```python
from build123d import *

# Parameters (mm, degrees)
EXTRUDE_START                           = -72
EXTRUDE_SKETCH_1_R                      = 82
EXTRUDE_SKETCH_1_R_2                    = 66
EXTRUDE_1_DEPTH                         = 12
EXTRUDE_START_2                         = -380
EXTRUDE_SKETCH_2_R                      = 3
EXTRUDE_2_DEPTH                         = 308
EXTRUDE_SKETCH_3_R                      = 3
EXTRUDE_3_DEPTH                         = 308
EXTRUDE_SKETCH_4_R                      = 3
EXTRUDE_4_DEPTH                         = 308
EXTRUDE_SKETCH_5_R                      = 3
EXTRUDE_5_DEPTH                         = 308
EXTRUDE_SKETCH_6_R                      = 3
EXTRUDE_6_DEPTH                         = 308
EXTRUDE_SKETCH_7_R                      = 3
EXTRUDE_7_DEPTH                         = 308
EXTRUDE_SKETCH_8_R                      = 3
EXTRUDE_8_DEPTH                         = 308
EXTRUDE_SKETCH_9_R                      = 3
EXTRUDE_9_DEPTH                         = 308
EXTRUDE_START_3                         = -170
EXTRUDE_SKETCH_10_R                     = 80
EXTRUDE_SKETCH_10_R_2                   = 70
EXTRUDE_10_DEPTH                        = 4
EXTRUDE_START_4                         = -275
EXTRUDE_SKETCH_11_R                     = 80
EXTRUDE_SKETCH_11_R_2                   = 70
EXTRUDE_11_DEPTH                        = 4
EXTRUDE_START_5                         = -384
EXTRUDE_SKETCH_12_R                     = 80
EXTRUDE_SKETCH_12_R_2                   = 64
EXTRUDE_12_DEPTH                        = 4
EXTRUDE_SKETCH_13_W                     = 129
EXTRUDE_SKETCH_13_H                     = 6
EXTRUDE_13_DEPTH                        = 4
EXTRUDE_SKETCH_14_W                     = 6
EXTRUDE_SKETCH_14_H                     = 61.49
EXTRUDE_14_DEPTH                        = 4
EXTRUDE_SKETCH_15_W                     = 6
EXTRUDE_SKETCH_15_H                     = 61.49
EXTRUDE_15_DEPTH                        = 4
COMBINE_START                           = -384
COMBINE_WELD_ASSEMBLY_OF_FEATURES_OUT_W = 6
COMBINE_WELD_ASSEMBLY_OF_FEATURES_OUT_H = 0.01
COMBINE_WELD_ASSEMBLY_OF_FEATURES_DEPTH = 4


# Read off the part's stored shape, not the designer's step: Combine _weld _ assembly of features_
with BuildPart() as part:
    # Extrude sketch 1 → Extrude 1 (new body)
    with BuildSketch(Plane.XY.offset(EXTRUDE_START)):
        with Locations((240, 0)):
            Circle(EXTRUDE_SKETCH_1_R)
        with Locations((240, 0)):
            Circle(EXTRUDE_SKETCH_1_R_2, mode=Mode.SUBTRACT)
    extrude(amount=EXTRUDE_1_DEPTH)


with BuildPart() as body_2:
    # Extrude sketch 2 → Extrude 2 (new body)
    with BuildSketch(Plane.XY.offset(EXTRUDE_START_2)):
        with Locations((308.367085406, 28.318573995)):
            Circle(EXTRUDE_SKETCH_2_R)
    extrude(amount=EXTRUDE_2_DEPTH)


with BuildPart() as body_3:
    # Extrude sketch 3 → Extrude 3 (new body)
    with BuildSketch(Plane.XY.offset(EXTRUDE_START_2)):
        with Locations((268.318573995, 68.367085406)):
            Circle(EXTRUDE_SKETCH_3_R)
    extrude(amount=EXTRUDE_3_DEPTH)


with BuildPart() as body_4:
    # Extrude sketch 4 → Extrude 4 (new body)
    with BuildSketch(Plane.XY.offset(EXTRUDE_START_2)):
        with Locations((211.681426005, 68.367085406)):
            Circle(EXTRUDE_SKETCH_4_R)
    extrude(amount=EXTRUDE_4_DEPTH)


with BuildPart() as body_5:
    # Extrude sketch 5 → Extrude 5 (new body)
    with BuildSketch(Plane.XY.offset(EXTRUDE_START_2)):
        with Locations((171.632914594, 28.318573995)):
            Circle(EXTRUDE_SKETCH_5_R)
    extrude(amount=EXTRUDE_5_DEPTH)


with BuildPart() as body_6:
    # Extrude sketch 6 → Extrude 6 (new body)
    with BuildSketch(Plane.XY.offset(EXTRUDE_START_2)):
        with Locations((171.632914594, -28.318573995)):
            Circle(EXTRUDE_SKETCH_6_R)
    extrude(amount=EXTRUDE_6_DEPTH)


with BuildPart() as body_7:
    # Extrude sketch 7 → Extrude 7 (new body)
    with BuildSketch(Plane.XY.offset(EXTRUDE_START_2)):
        with Locations((211.681426005, -68.367085406)):
            Circle(EXTRUDE_SKETCH_7_R)
    extrude(amount=EXTRUDE_7_DEPTH)



with BuildPart() as body_8:
    # Extrude sketch 8 → Extrude 8 (new body)
    with BuildSketch(Plane.XY.offset(EXTRUDE_START_2)):
        with Locations((268.318573995, -68.367085406)):
            Circle(EXTRUDE_SKETCH_8_R)
    extrude(amount=EXTRUDE_8_DEPTH)


with BuildPart() as body_9:
    # Extrude sketch 9 → Extrude 9 (new body)
    with BuildSketch(Plane.XY.offset(EXTRUDE_START_2)):
        with Locations((308.367085406, -28.318573995)):
            Circle(EXTRUDE_SKETCH_9_R)
    extrude(amount=EXTRUDE_9_DEPTH)


with BuildPart() as body_10:
    # Extrude sketch 10 → Extrude 10 (new body)
    with BuildSketch(Plane.XY.offset(EXTRUDE_START_3)):
        with Locations((240, 0)):
            Circle(EXTRUDE_SKETCH_10_R)
        with Locations((240, 0)):
            Circle(EXTRUDE_SKETCH_10_R_2, mode=Mode.SUBTRACT)
    extrude(amount=EXTRUDE_10_DEPTH)


with BuildPart() as body_11:
    # Extrude sketch 11 → Extrude 11 (new body)
    with BuildSketch(Plane.XY.offset(EXTRUDE_START_4)):
        with Locations((240, 0)):
            Circle(EXTRUDE_SKETCH_11_R)
        with Locations((240, 0)):
            Circle(EXTRUDE_SKETCH_11_R_2, mode=Mode.SUBTRACT)
    extrude(amount=EXTRUDE_11_DEPTH)


with BuildPart() as body_12:
    # Extrude sketch 12 → Extrude 12 (new body)
    with BuildSketch(Plane.XY.offset(EXTRUDE_START_5)):
        with Locations((240, 0)):
            Circle(EXTRUDE_SKETCH_12_R)
        with Locations((240, 0)):
            Circle(EXTRUDE_SKETCH_12_R_2, mode=Mode.SUBTRACT)
    extrude(amount=EXTRUDE_12_DEPTH)


with BuildPart() as body_13:
    # Extrude sketch 13 → Extrude 13 (new body)
    with BuildSketch(Plane.XY.offset(EXTRUDE_START_5)):
        with Locations((240, 0)):
            Rectangle(EXTRUDE_SKETCH_13_W, EXTRUDE_SKETCH_13_H)
    extrude(amount=EXTRUDE_13_DEPTH)


with BuildPart() as body_14:
    # Extrude sketch 14 → Extrude 14 (new body)
    with BuildSketch(Plane.XY.offset(EXTRUDE_START_5)):
        with Locations((240, -33.755)):
            Rectangle(EXTRUDE_SKETCH_14_W, EXTRUDE_SKETCH_14_H)
    extrude(amount=EXTRUDE_14_DEPTH)


with BuildPart() as body_15:
    # Extrude sketch 15 → Extrude 15 (new body)
    with BuildSketch(Plane.XY.offset(EXTRUDE_START_5)):
        with Locations((240, 33.755)):
            Rectangle(EXTRUDE_SKETCH_15_W, EXTRUDE_SKETCH_15_H)
    extrude(amount=EXTRUDE_15_DEPTH)


with BuildPart() as body_7_1:
    add(body_7.part)

    add(body_14.part)  # Combine _weld _ assembly of features merges body 14

    add(body_10.part)  # Combine _weld _ assembly of features merges body 10

    add(body_9.part)  # Combine _weld _ assembly of features merges body 9

    add(body_11.part)  # Combine _weld _ assembly of features merges body 11

    add(part.part)  # Combine _weld _ assembly of features merges part

    add(body_2.part)  # Combine _weld _ assembly of features merges body 2

    add(body_12.part)  # Combine _weld _ assembly of features merges body 12

    add(body_8.part)  # Combine _weld _ assembly of features merges body 8

    add(body_13.part)  # Combine _weld _ assembly of features merges body 13

    add(body_5.part)  # Combine _weld _ assembly of features merges body 5

    add(body_4.part)  # Combine _weld _ assembly of features merges body 4

    add(body_6.part)  # Combine _weld _ assembly of features merges body 6

    add(body_15.part)  # Combine _weld _ assembly of features merges body 15

    add(body_3.part)  # Combine _weld _ assembly of features merges body 3
    # Combine _weld _ assembly of features out → Combine _weld _ assembly of features (add)
    with BuildSketch(Plane.XY.offset(COMBINE_START)):
        with Locations((240, 3.005)):
            Rectangle(COMBINE_WELD_ASSEMBLY_OF_FEATURES_OUT_W, COMBINE_WELD_ASSEMBLY_OF_FEATURES_OUT_H)
        with Locations((240, -3.005)):
            Rectangle(COMBINE_WELD_ASSEMBLY_OF_FEATURES_OUT_W, COMBINE_WELD_ASSEMBLY_OF_FEATURES_OUT_H)
    extrude(amount=COMBINE_WELD_ASSEMBLY_OF_FEATURES_DEPTH)


solid = body_7_1.part
```
Design review of the part built by this model. Coordinates are the model's own, in mm. A direction names the side the tool comes from. Round coordinates to 2 decimals unless told otherwise and drop trailing zeros. Write each loop counter-clockwise with the first axis right and the second up, starting at its lowest first coordinate (ties: lowest second). Pieces come first, ordered by that corner, then holes. Notation, with made-up numbers: (-6.75, -38.75) -> (3.25, -38.75) arc R20 cw to (3.25, -9.75) -> close; hole circle Ø10 at (-5.75, 30.25). An arc over 180 degrees is marked (long way). Answer in a Markdown table with one row per item.
Q1. For faces 4 (the face through (173.02, 25.66, -221.21)), 5 (the face through (174.064, 2.902, -66.084)), 6 (the face through (194.28, -44.785, -382.028)), list the 3-axis set-ups (+Z, -Z, +X, -X, +Y, -Y) from which the entire face can be reached by the end or side of a thin tool; tool diameter is ignored.
The answers:
| item | result |
|---|---|
| face 4 | none |
| face 5 | +Z |
| face 6 | +Z, -Z |
Q2. Take a section at A-A, the plane z = -315.5. State the section outline as (x, y) points.
The answers:
| item | result |
|---|---|
| outline | circle Ø6 at (171.63, -28.32); circle Ø6 at (171.63, 28.32); circle Ø6 at (211.68, -68.37); circle Ø6 at (211.68, 68.37); circle Ø6 at (268.32, -68.37); circle Ø6 at (268.32, 68.37); circle Ø6 at (308.37, -28.32); circle Ø6 at (308.37, 28.32) |
Q3. To check wall thickness, follow L1, parallel to Z at x = 273.5, y = 71.5; L2, parallel to Y at x = 240, z = -167; L3, parallel to Y at x = 240, z = -65.25. State the ranges of each line that lie inside material, in increasing order. Write a range as [from, to].
The answers:
| item | result |
|---|---|
| L1 | [-384, -380], [-275, -271], [-170, -166], [-72, -60] |
| L2 | [-80, -70], [70, 80] |
| L3 | [-82, -66], [66, 82] |
Q4. Take a section at B-B, the plane y = -17.5. Count the separate pieces of the cut face and the enclosed holes in it, then the cut area to 3 significant figures.
The answers:
| item | result |
|---|---|
| separate pieces | 9 |
| enclosed holes | 0 |
| area | 716 mm² |
Q5. Draft analysis for pull direction X (two halves, no side actions). For faces 1 (the face through (195.215, 45.72, -382.028)), 2 (the face through (239, 1, -384)), 3 (the face through (316.306, 24.03, -382.028)), state which applies: +X half, -X half, draft (parallel to the pull), parting line (faces both ways), or undercut.
The answers:
| item | result |
|---|---|
| face 1 | undercut |
| face 2 | draft |
| face 3 | parting line |
Q6. Clearance check with flat-ended pins moving along their axes: pin 1 Ø4.5 at (x, z) = (263, -382.5) entering from +Y; pin 2 Ø3 at (y, z) = (38, -382) entering from -X; pin 3 Ø1 at (x, z) = (209.5, -221.5) entering from +Y. State where each tip first meets the part, or that it passes through.
The answers:
| item | result |
|---|---|
| pin 1 | y = 77.26 |
| pin 2 | x = 168.81 |
| pin 3 | y = 70.85 |
